Can you work these out from the drawing? Everything is in mm from the part's minimum corner. A direction names the side the tool comes from. Coordinates: 2 decimals unless noted, no trailing zeros. Order: outer loops, then holes, each group sorted by start corner. A loop starts at its lowest first (then second) coordinate and runs counter-clockwise, first axis right, second up. Notation, with made-up numbers: M 18.5,40 L 66.5,40 A11 cw 66.5,44 Z; hole C 56.5,64 d10. An arc over 180 degrees is marked long. Answer as a JSON object with one key per item and string values.
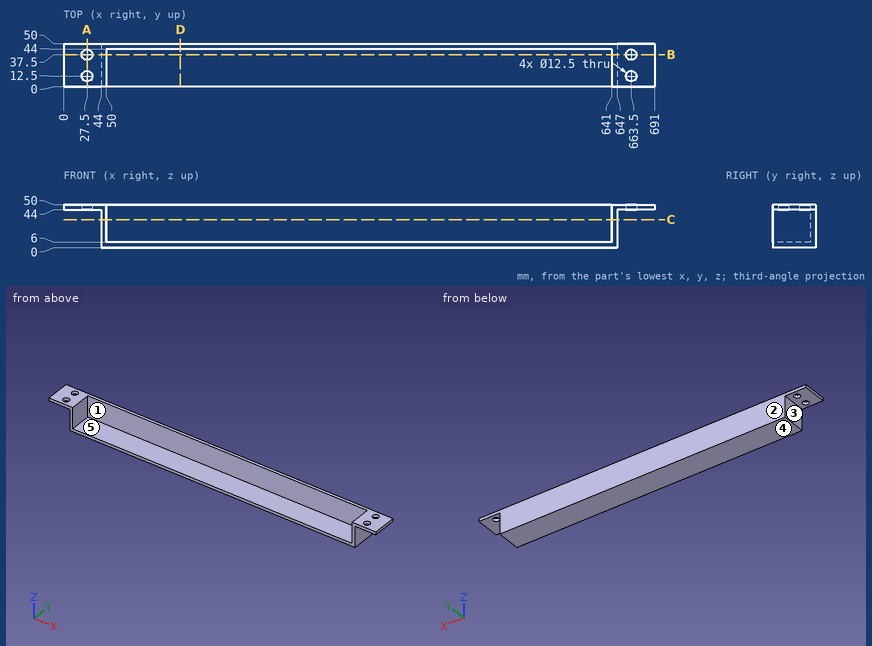
Item 1: I want a section at B-B, the plane y = 37.5. Write out the boundary of the cut face in (x, z), plus the area to 3 significant figures.
Answers follow:
{"outline": "M 0,44 L 21.25,44 L 21.25,50 L 0,50 Z; M 33.75,44 L 44,44 L 44,0 L 647,0 L 647,44 L 657.25,44 L 657.25,50 L 641,50 L 641,6 L 50,6 L 50,50 L 33.75,50 Z; M 669.75,44 L 691,44 L 691,50 L 669.75,50 Z", "area": "4,520 mm^2"}
Item 2: I want a section at D-D, the plane x = 136.5. Write out the boundary of the cut face in (y, z).
Answers follow:
{"outline": "M 0,0 L 50,0 L 50,50 L 44,50 L 44,6 L 0,6 Z"}
Item 3: I'm going to push flat-ended pins straight in: pin 1 (7.5 mm diameter, centred on x = 663.5, y = 37.5, fed in from +Z); pin 2 (22 mm diameter, centred on x = 400, z = 32, fed in from -Y); pin 3 (13 mm diameter, centred on y = 25.5, z = 28, fed in from -X); pin 4 (8 mm diameter, centred on x = 413.5, y = 14.5, fed in from +Z). Where does each tip first touch, or does it pass through?
Answers follow:
{"pin 1": "passes through", "pin 2": "stops at y = 44", "pin 3": "stops at x = 44", "pin 4": "stops at z = 6"}
Item 4: Which directions (+Z, -Z, +X, -X, +Y, -Y) give clear straight access to the entire face, cutting with the end or side of a thin tool? Please do the marked faces 4 and 5.
Answers follow:
{"face 4": "-Z, +X, -X, +Y, -Y", "face 5": "+Z, -Y"}
Item 5: I want a section at C-C, the plane z = 32.5. Write out the boundary of the cut face in (x, y), plus the area to 3 significant figures.
Answers follow:
{"outline": "M 44,0 L 50,0 L 50,44 L 641,44 L 641,0 L 647,0 L 647,50 L 44,50 Z", "area": "4,150 mm^2"}
Item 6: Please list where these lines run through material, in increasing order: line 1 (X direction, y = 37, z = 47); line 2 (Y direction, x = 27.5, z = 46.9); line 3 (X direction, y = 24, z = 32).
Answers follow:
{"line 1": "x = 0 to 21.27, 33.73 to 50, 641 to 657.27, 669.73 to 691", "line 2": "y = 0 to 6.25, 18.75 to 31.25, 43.75 to 50", "line 3": "x = 44 to 50, 641 to 647"}
Item 7: I want a section at A-A, the plane x = 27.5. Write out the boundary of the cut face in (y, z), plus the area to 3 significant figures.
Answers follow:
{"outline": "M 0,44 L 6.25,44 L 6.25,50 L 0,50 Z; M 18.75,44 L 31.25,44 L 31.25,50 L 18.75,50 Z; M 43.75,44 L 50,44 L 50,50 L 43.75,50 Z", "area": "150 mm^2"}
Item 8: If we mould it in two halves opening along X, with no side actions, what happens to the marked faces 1, 2 and 3? For each: pulls with the +X half, pulls with the -X half, needs draft (parallel to the pull), parting line crosses it, or undercut.
Answers follow:
{"face 1": "undercut", "face 2": "needs draft", "face 3": "pulls with the -X half"}
